from build123d import *

# Parameters (mm, degrees)
SKETCH1_W                = 8
SKETCH1_H                = 12
BOSS_EXTRUDE1_DEPTH      = 2.1
SKETCH2_W                = 2
SKETCH2_H                = 6
CUT_EXTRUDE1_DEPTH       = 2.1
CUT_EXTRUDE4_START       = -12
CUT_EXTRUDE4_DEPTH       = 12
SKETCH4_W                = 6
SKETCH4_H                = 1.1
CUT_EXTRUDE5_DEPTH       = 0.5
CUT_EXTRUDE14_DEPTH      = 6
FILLET1_R                = 1
FILLET2_R                = 0.4
CUT_EXTRUDE15_DEPTH      = 15.574292436
CUT_EXTRUDE15_DEPTH_BACK = 15.574292436
SKETCH8_R                = 0.3
CUT_EXTRUDE16_DEPTH      = 15.574292587
SKETCH9_R                = 0.3
CUT_EXTRUDE17_DEPTH      = 10
FILLET4_R                = 0.8


# Read off the part's stored shape, not the designer's step: Cut-Extrude4
with BuildPart() as part:
    # Sketch1 → Boss-Extrude1 (new body)
    with BuildSketch(Plane(origin=(0, 0, 0), x_dir=(1, 0, 0), z_dir=(0, 1, 0))):
        with Locations((4, 6)):
            Rectangle(SKETCH1_W, SKETCH1_H)
    extrude(amount=BOSS_EXTRUDE1_DEPTH)

    # Sketch2 → Cut-Extrude1 (cut)
    with BuildSketch(Plane(origin=(0, 2.1, 0), x_dir=(1, 0, 0), z_dir=(0, 1, 0))):
        with Locations((7, 6)):
            Rectangle(SKETCH2_W, SKETCH2_H)
    extrude(amount=-CUT_EXTRUDE1_DEPTH, mode=Mode.SUBTRACT)

    # Cut-Extrude4 outline → Cut-Extrude4 (cut)
    with BuildSketch(Plane.XY.offset(CUT_EXTRUDE4_START)):
        with BuildLine():
            ThreePointArc((5.744749223, 1), (5.817245121, 1.031120796), (5.844618418, 1.105113104))
            Line((5.844618418, 1.105113104), (5.793682188, 2.1))
            Line((5.793682188, 2.1), (4.513567693, 2.1))
            Line((4.513567693, 2.1), (4.45611228, 1.105769256))
            ThreePointArc((4.45611228, 1.105769256), (4.483223902, 1.031359362), (4.555945719, 1))
            Line((4.555945719, 1), (5.744749223, 1))
        make_face()
    extrude(amount=CUT_EXTRUDE4_DEPTH, mode=Mode.SUBTRACT)

    # Sketch4 → Cut-Extrude5 (cut)
    with BuildSketch(Plane(origin=(6, 0, 0), x_dir=(0, 0, -1), z_dir=(1, 0, 0))):
        with Locations((6, 1.55)):
            Rectangle(SKETCH4_W, SKETCH4_H)
    extrude(amount=-CUT_EXTRUDE5_DEPTH, mode=Mode.SUBTRACT)

    # Sketch6 → Cut-Extrude14 (cut)
    with BuildSketch(Plane.XY.offset(-9)):
        Polygon((6, 0), (6, 1), (5.619051105, 1), align=None)
    extrude(amount=CUT_EXTRUDE14_DEPTH, mode=Mode.SUBTRACT)

    # Fillet1
    fillet1_edges = [part.edges().sort_by_distance(p)[0] for p in [
        (0, 2.1, -6),
        (0, 0, -6),
    ]]
    fillet(fillet1_edges, radius=FILLET1_R)

    # Fillet2
    fillet2_edges = [part.edges().sort_by_distance(p)[0] for p in [
        (8, 0, -10.5),
        (8, 0, -1.5),
    ]]
    fillet(fillet2_edges, radius=FILLET2_R)

    # Sketch7 → Cut-Extrude15 (cut, two sides: drawn at the far end of the back side and taken through both)
    with BuildSketch(Plane.XY.offset(-CUT_EXTRUDE15_DEPTH_BACK)):
        with BuildLine():
            Line((8, 2.1), (6.963365026, 2.1))
            add(Edge.make_bspline(
                [(6.963365026, 2.1), (7.9845252, 1.726197455), (8, 0.549529298)],
                knots=[0, 0, 0, 0.970144169, 0.970144169, 0.970144169], degree=2))
            Line((8, 0.549529298), (8, 2.1))
        make_face()
    extrude(amount=CUT_EXTRUDE15_DEPTH + CUT_EXTRUDE15_DEPTH_BACK, mode=Mode.SUBTRACT)

    # Sketch8 → Cut-Extrude16 (cut, through all)
    with BuildSketch(Plane.XY):
        with Locations((1.25, 1.05)):
            Circle(SKETCH8_R)
    extrude(amount=-CUT_EXTRUDE16_DEPTH, mode=Mode.SUBTRACT)

    # Sketch9 → Cut-Extrude17 (cut)
    with BuildSketch(Plane(origin=(0, 0, -12), x_dir=(-1, 0, 0), z_dir=(0, 0, -1))):
        with Locations((-6.75, 0.9)):
            Circle(SKETCH9_R)
    extrude(amount=-CUT_EXTRUDE17_DEPTH, mode=Mode.SUBTRACT)

    # Fillet4
    fillet4_edges = [part.edges().sort_by_distance(p)[0] for p in [
        (6.963365026, 2.1, -10.5),
        (6.963365026, 2.1, -1.5),
    ]]
    fillet(fillet4_edges, radius=FILLET4_R)


solid = part.part
Read the model definition and answer for the solid it produces. Units are mm, in the model's axes. A direction names the side the tool comes from. Give positions to 0.01 mm unless a question says otherwise; leave off trailing zeros. Write each loop counter-clockwise with the first axis right and the second up, starting at its lowest first coordinate (ties: lowest second). Pieces come first, ordered by that corner, then holes. Notation, with made-up numbers: M 74.25,8.5 L 109.25,8.5 A23 cw 109.25,21.5 Z; hole C 27.25,-39 d11. An arc over 180 degrees is marked long. One line per item, written item: value. Start each with the question number.
(1) Find the intervals of material crossed by line 1 (Y direction, x = 6.75, z = -10.9); line 2 (Z direction, x = 6, y = 0.1); line 3 (X direction, y = 0.85, z = -11.25), in increasing order.
(2) Find section D-D (x = 5.5). Determine the outline of the cut face in (y, z), plus the area to 3 significant figures.
(3) Flat-ended cylindrical pins translate along their axes: pin 1 Ø4 at (x, z) = (5.5, -2) entering from +Y; pin 2 Ø1 at (x, z) = (5.5, -3.5) entering from +Y. Find the tip coordinate at first contact, or state that the pin passes through.
(4) Find section A-A (x = 1.25). Determine the outline of the cut face in (y, z).
(5) Determine the mould class of faces 6 (the flat face through (7.1, 1.3, -3)), 7 (the flat face through (7.1, 1.3, -9)), 8 (the flat face through (5.82, 1.6, -1.52)), 9 (the flat face through (4, 1, 0)) for opening direction Z: pulls with the +Z half, pulls with the -Z half, needs draft (parallel to the pull), parting line crosses it, or undercut.
(6) Find section C-C (y = 1.7). Give the number of separate pieces and of enclosed holes in the cut face, plus the area to 3 significant figures.
(7) Find section B-B (z = -6). Determine the outline of the cut face in (x, y), plus the area to 3 significant figures.
(8) A tool of negligible diameter and unlimited length cuts with its end or side. For faces 1 (the flat face through (5.82, 1.6, -10.52)), 2 (the flat face through (4, 1, -12)), 3 (the flat face through (5, 1, -6)), 4 (the flat face through (6, 2.1, -2)), 5 (the flat face through (5.807, 0.507, -6.042)), from which of +Z, -Z, +X, -X, +Y, -Y can it reach the whole face along a straight path? Write none if from no direction.
Results below:
1. line 1: y = 0 to 0.6, 1.2 to 2.1
1. line 2: z = -12 to -9, -3 to 0
1. line 3: x = 0.01 to 1.03, 1.47 to 6.45, 7.05 to 7.98
2. outline: M 0,-12 L 1,-12 L 1,0 L 0,0 Z
2. area: 12.0 mm^2
3. pin 1: stops at y = 2.1
3. pin 2: stops at y = 1
4. outline: M 0,-12 L 0.75,-12 L 0.75,0 L 0,0 Z; M 1.35,-12 L 2.1,-12 L 2.1,0 L 1.35,0 Z
5. face 6: undercut
5. face 7: undercut
5. face 8: needs draft
5. face 9: pulls with the +Z half
6. separate pieces: 3
6. enclosed holes: 0
6. area: 62.2 mm^2
7. outline: M 0,1 A1 ccw 1,0 L 6,0 L 5.62,1 L 4.56,1 A0.1 cw 4.46,1.11 L 4.51,2.1 L 1,2.1 A1 ccw 0,1.1 Z; hole C 1.25,1.05 d0.6
7. area: 10.0 mm^2
8. face 1: +Z, -Z
8. face 2: -Z, +X, -X, +Y, -Y
8. face 3: +Z, -Z, +Y
8. face 4: +Z, -Z, +X, -X, +Y
8. face 5: +X, +Y
